Geometry: see drawing. Coordinates: mm, zero at the bounding-box minimum. A direction names the side the tool comes from. Give positions to 0.01 mm unless a question says otherwise; leave off trailing zeros. Write each loop counter-clockwise with the first axis right and the second up, starting at its lowest first coordinate (ties: lowest second). Pieces come first, ordered by that corner, then holes. Notation, with made-up numbers: M 7.25,39 L 20.25,39 A14 cw 20.25,49 Z; hole C 2.5,56.5 d1. An arc over 180 degrees is marked long. Use one line per item in the form item = value. Start each with the question number.
Item 1: Section query B-B on x = 5. Return loops of the section in (y, z), then the cut area to 3 significant figures.
Item 2: Material intervals for line 1 along Y through (x, z) = (6, 1.75); line 2 along X through (y, z) = (23.5, 1); line 3 along Z through (x, y) = (3.5, 12), sorted ascending. Write a range as from..to.
Item 3: Section query C-C on y = 4. Return loops of the section in (x, z).
Item 4: Contact query for flat-ended pins moving along their axis: P1, Ø1, axis at x = 7.5, y = 6.5, coming from the -Z side; P2, Ø6, axis at x = 6, y = 6, coming from the +Z side; P3, Ø6, axis at y = 4.5, z = 5.5, coming from the -X side. Output: stop coordinate, or through.
Item 5: Section query A-A on z = 5. Return loops of the section in (x, y), then the cut area to 3 significant figures.
Item 6: Access query for the marked faces 1 and 2. Directions: +Z, -Z, +X, -X, +Y, -Y. A direction counts if a zero-diameter tool reaches every point of the face in a straight line with its end or side. Return the directions, or none.
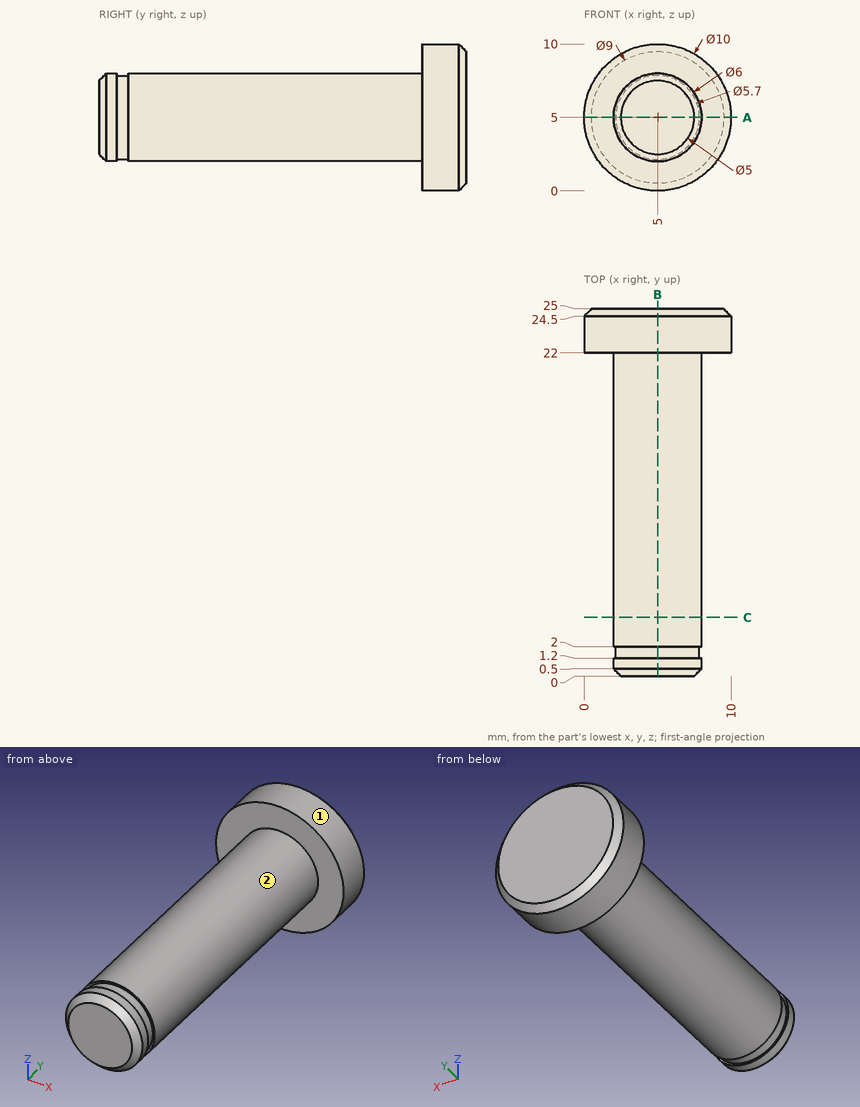
Answer sheet:
q1.outline = M 0,2.5 L 0.5,2 L 1.2,2 L 1.2,2.15 L 2,2.15 L 2,2 L 22,2 L 22,0 L 24.5,0 L 25,0.5 L 25,9.5 L 24.5,10 L 22,10 L 22,8 L 2,8 L 2,7.85 L 1.2,7.85 L 1.2,8 L 0.5,8 L 0,7.5 Z
q1.area = 161 mm2
q2.line_1 = 22..25
q2.line_2 = 2..8
q2.line_3 = 2.4..7.6
q3.outline = C 5,5 d6
q4.P1 = 2.76
q4.P2 = 8
q4.P3 = 2
q5.outline = M 0,22 L 2,22 L 2,2 L 2.15,2 L 2.15,1.2 L 2,1.2 L 2,0.5 L 2.5,0 L 7.5,0 L 8,0.5 L 8,1.2 L 7.85,1.2 L 7.85,2 L 8,2 L 8,22 L 10,22 L 10,24.5 L 9.5,25 L 0.5,25 L 0,24.5 Z
q5.area = 161 mm2
q6.face_1 = +Y, -Y
q6.face_2 = -Y
